CAD build for the part. Positions are in the model's coordinates, mm. A direction names the side the tool comes from. Give positions to 0.01 mm unless a question says otherwise; leave off trailing zeros. Write each loop counter-clockwise with the first axis right and the second up, starting at its lowest first coordinate (ties: lowest second). Pieces come first, ordered by that corner, then holes. Notation, with made-up numbers: (50.25, -14) - (99.25, -14) arc R25 cw to (99.25, 22) - close; hole circle Ø7 at (35.5, 86). An arc over 180 degrees is marked (long way). Answer as a JSON object with one key per item and string values.
from build123d import *

# Parameters (mm, degrees)
F0_W           = 45
F0_H           = 25
F1_DEPTH       = 6
F2_R           = 5
F4_R           = 5.5
F5_DEPTH       = 25
F6_R           = 2.1
F7_DEPTH       = 25
F9_R           = 7.5
F10_DEPTH      = 5
F10_DEPTH_BACK = 25
F11_W          = 49.2877000943
F11_H          = 30.2235903218
F12_DEPTH      = 25
F13_W          = 37.6632460393
F13_H          = 10.6945014559
F14_DEPTH      = 25
F15_R          = 3
F16_DEPTH      = 25
F16_DEPTH_BACK = 25
F18_R          = 3


# Not quite as in the source:
# - a fillet or chamfer that OpenCascade refuses, or shapes differently, is made with other operations: its cross-section is extruded or revolved along the edge and cut away or added


with BuildPart() as f1:
    # F0 (on Top) → F1 (new body)
    with BuildSketch(Plane.XY):
        with Locations((22.5, 12.5)):
            Rectangle(F0_W, F0_H)
    extrude(amount=F1_DEPTH)

    # F2
    f2_edges = [f1.edges().sort_by_distance(p)[0] for p in [
        (45, 25, 3),
        (45, 0, 3),
        (0, 25, 3),
        (0, 0, 3),
    ]]
    fillet(f2_edges, radius=F2_R)

    # F4 (on offset) → F5 (cut)
    with BuildSketch(Plane.XY.offset(5)):
        with Locations((6.75, 12.5)):
            Circle(F4_R)
        with Locations((38.25, 12.5)):
            Circle(F4_R)
    extrude(amount=F5_DEPTH, mode=Mode.SUBTRACT)

    # F6 (on Top) → F7 (cut)
    with BuildSketch(Plane.XY):
        with Locations((6.75, 12.5)):
            Circle(F6_R)
        with Locations((38.25, 12.5)):
            Circle(F6_R)
    extrude(amount=F7_DEPTH, mode=Mode.SUBTRACT)

    # F9 (on face) → F10 (join, two sides)
    with BuildSketch(Plane(origin=(0, -2.954423259, 2.479055467), x_dir=(1, 0, 0), z_dir=(0, -0.7660444431, 0.6427876097))) as f10_sk:
        with Locations((22.5, 8)):
            Circle(F9_R)
    extrude(amount=F10_DEPTH)
    extrude(f10_sk.sketch, amount=-F10_DEPTH_BACK)

    # F11 (on Top) → F12 (cut)
    with BuildSketch(Plane.XY):
        with Locations((22.6797270589, 13.7661970221)):
            Rectangle(F11_W, F11_H)
    extrude(amount=-F12_DEPTH, mode=Mode.SUBTRACT)

    # F13 (on face) → F14 (cut)
    with BuildSketch(Plane(origin=(0, 25, 0), x_dir=(-1, 0, 0), z_dir=(0, 1, 0))):
        with Locations((-22.6992729586, 2.3689556401)):
            Rectangle(F13_W, F13_H)
    extrude(amount=F14_DEPTH, mode=Mode.SUBTRACT)

    # F15 (on face) → F16 (cut, two sides)
    with BuildSketch(Plane(origin=(0, -2.954423259, 2.479055467), x_dir=(1, 0, 0), z_dir=(0, -0.7660444431, 0.6427876097))) as f16_sk:
        with Locations((22.5, 8)):
            Circle(F15_R)
    extrude(amount=F16_DEPTH, mode=Mode.SUBTRACT)
    extrude(f16_sk.sketch, amount=-F16_DEPTH_BACK, mode=Mode.SUBTRACT)

    # F17: chamfer of 3 x 5 on 1 edges, made by hand

    # F17_s1 → F17_t2 (revolve, cut)
    with BuildSketch(Plane(origin=(0, 5.1423008775, 6.128355545), x_dir=(1, 0, 0), z_dir=(0, 0.6427876097, 0.7660444431))):
        Polygon((28.5, -8.8567256581), (25.5, -3.8567256581), (25.5, -8.8567256581), align=None)
    revolve(axis=Axis((22.5, -1.6423445971, 11.8213490604), (0, 0.7660444431, -0.6427876097)), mode=Mode.SUBTRACT)

    # F18
    f18_edges = [f1.edges().sort_by_distance(p)[0] for p in [
        (19.5, 2.187878, 8.607411),
    ]]
    fillet(f18_edges, radius=F18_R)

    # F19: fillet of radius 3 on 1 edges, made by hand

    # F19_s1 → F19_t2 (revolve, cut)
    with BuildSketch(Plane(origin=(0, 5.1423008775, 6.128355545), x_dir=(1, 0, 0), z_dir=(0, 0.6427876097, 0.7660444431))):
        with BuildLine():
            ThreePointArc((27.6302051352, -7.4070675501), (28.6371938466, -8.4227287465), (30, -8.8567256581))
            Line((30, -8.8567256581), (28.5, -8.8567256581))
            Line((28.5, -8.8567256581), (27.6302051352, -7.4070675501))
        make_face()
    revolve(axis=Axis((22.5, -1.6423445971, 11.8213490604), (0, 0.7660444431, -0.6427876097)), mode=Mode.SUBTRACT)


solid = f1.part
(1) Flat gauge pins, fed straight in: P1, Ø9, axis at x = 37.5, y = 10, coming from the +Z side; P2, Ø10, axis at x = 30.5, y = 4.5, coming from the -Z side; P3, Ø6.5, axis at x = 38.25, y = 12.5, coming from the +Z side; P4, Ø7.5, axis at x = 28, y = 11.5, coming from the +Z side. Where does each tip first touch, or does it go through?
Answer key:
{"P1": "stops at z = 6", "P2": "stops at z = 0", "P3": "stops at z = 5", "P4": "stops at z = 12.13"}
(2) Saw through at A-A, the plane x = 38.25. Give the cut face in (y, z), and give its area (3 significant figures).
Answer key:
{"outline": "(0, 0) - (10.4, 0) - (10.4, 5) - (7, 5) - (7, 6) - (0, 6) - close; (14.6, 0) - (25, 0) - (25, 6) - (18, 6) - (18, 5) - (14.6, 5) - close", "area": "118 mm²"}
(3) Pull direction X, two halves, no side cores. Call faces 3 (the face through (0, 12, 3)), 4 (the face through (22.11, 9.46, 6.39)), 5 (the face through (22, 18, 6)): pulls with the +X half, pulls with the -X half, needs draft (parallel to the pull), parting line crosses it, or undercut.
Answer key:
{"face 3": "pulls with the -X half", "face 4": "undercut", "face 5": "needs draft"}
(4) Saw through at B-B, the plane y = 13.5. State how many separate pieces and enclosed holes the cut face has, and give its area (3 significant figures).
Answer key:
{"separate pieces": "3", "enclosed holes": "0", "area": "220 mm²"}
(5) Probe L1, parallel to X at y = 12.5, z = 5.65; L2, parallel to Y at x = 6.75, z = 2.65; L3, parallel to Y at x = 6.75, z = 5.7. List the from-to ranges inside material, lowest first. Write a range as [from, to].
Answer key:
{"L1": "x = [0, 1.25], [12.25, 32.75], [43.75, 45]", "L2": "y = [0, 10.4], [14.6, 25]", "L3": "y = [0, 7], [18, 25]"}
(6) 3-axis set-ups, long thin cutter, end or side, ignore diameter. For faces 1 (the face through (9, 13, 5)), 2 (the face through (1, 2, 3)): which of +Z, -Z, +X, -X, +Y, -Y reach the whole face in a straight line?
Answer key:
{"face 1": "+Z", "face 2": "+Z, -Z, -X, -Y"}
(7) Saw through at C-C, the plane x = 7.5. Give the cut face in (y, z), and give its area (3 significant figures).
Answer key:
{"outline": "(0, 0) - (10.54, 0) - (10.54, 5) - (7.05, 5) - (7.05, 6) - (0, 6) - close; (14.46, 0) - (25, 0) - (25, 6) - (17.95, 6) - (17.95, 5) - (14.46, 5) - close", "area": "119 mm²"}
